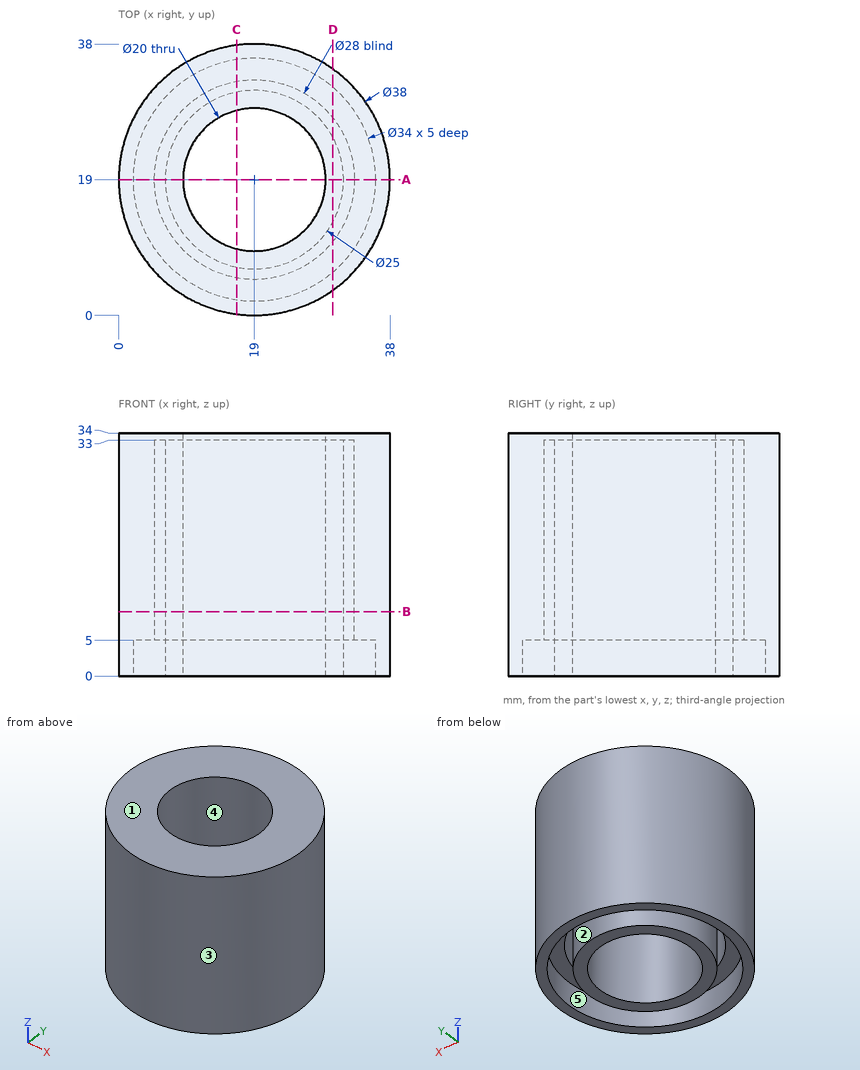
Drawing for the job (mm, zero at the part's lowest x, y, z). A direction names the side the tool comes from. Coordinates: 2 decimals unless noted, no trailing zeros. Order: outer loops, then holes, each group sorted by start corner. A loop starts at its lowest first (then second) coordinate and runs counter-clockwise, first axis right, second up. Notation, with made-up numbers: (-17.75, 64.25) - (29.25, 64.25) arc R36 ccw to (29.25, 102.25) - close; hole circle Ø10 at (-18.5, 9). An arc over 180 degrees is marked (long way). Use a Markdown table: item, result. Add a question column.
(1) Drill centre lines: line 1 along Y through (x, z) = (19, 10); line 2 along Y through (x, z) = (12, 24); line 3 along X through (y, z) = (23, 22). Where is each one in solid material? Low to high. Write a range as [from, to].
(2) Which spindle directions (+Z, -Z, +X, -X, +Y, -Y) get a long thin tool onto all of the face, cutting with end or side? Do the marked faces 4 and 5. Say none if no direction does.
(3) Saw through at D-D (x = 30). Give the cut face in (y, z).
(4) Saw through at C-C (x = 16.5). Give the cut face in (y, z), then the cut area to 3 significant figures.
(5) Pull direction Y, two halves, no side cores. Call the marked faces 1, 2 and 3: +Y half, -Y half, draft (parallel to the pull), parting line (faces both ways), or undercut.
(6) Flat gauge pins, fed straight in: pin 1 (1.5 mm diameter, centred on y = 15.5, z = 24.5, fed in from -X); pin 2 (5 mm diameter, centred on y = 8, z = 19.5, fed in from -X); pin 3 (5 mm diameter, centred on y = 10, z = 9.5, fed in from +X). Where does each tip first touch, or does it go through?
(7) Saw through at B-B (z = 9). Give the cut face in (x, y), then the cut area to 3 significant figures.
(8) Saw through at A-A (y = 19). Give the cut face in (x, z).
Solved:
| question | item | result |
|---|---|---|
| 1 | line 1 | y = [0, 5], [6.5, 9], [29, 31.5], [33, 38] |
| 1 | line 2 | y = [1.34, 6.88], [8.64, 11.86], [26.14, 29.36], [31.12, 36.66] |
| 1 | line 3 | x = [0.43, 5.58], [7.16, 9.83], [28.17, 30.84], [32.42, 37.57] |
| 2 | face 4 | +Z, -Z |
| 2 | face 5 | -Z |
| 3 | outline | (3.51, 0) - (6.04, 0) - (6.04, 5) - (10.34, 5) - (10.34, 33) - (13.06, 33) - (13.06, 0) - (24.94, 0) - (24.94, 33) - (27.66, 33) - (27.66, 5) - (31.96, 5) - (31.96, 0) - (34.49, 0) - (34.49, 34) - (3.51, 34) - close |
| 4 | outline | (0.17, 0) - (2.18, 0) - (2.18, 5) - (5.23, 5) - (5.23, 33) - (6.75, 33) - (6.75, 0) - (9.32, 0) - (9.32, 34) - (0.17, 34) - close; (28.68, 0) - (31.25, 0) - (31.25, 33) - (32.77, 33) - (32.77, 5) - (35.82, 5) - (35.82, 0) - (37.83, 0) - (37.83, 34) - (28.68, 34) - close |
| 4 | area | 491 mm² |
| 5 | face 1 | draft |
| 5 | face 2 | undercut |
| 5 | face 3 | parting line |
| 6 | pin 1 | stops at x = 0.2 |
| 6 | pin 2 | stops at x = 2.01 |
| 6 | pin 3 | stops at x = 36.85 |
| 7 | outline | circle Ø38 at (19, 19); circle Ø25 at (19, 19); hole circle Ø28 at (19, 19); hole circle Ø20 at (19, 19) |
| 7 | area | 695 mm² |
| 8 | outline | (0, 0) - (2, 0) - (2, 5) - (5, 5) - (5, 33) - (6.5, 33) - (6.5, 0) - (9, 0) - (9, 34) - (0, 34) - close; (29, 0) - (31.5, 0) - (31.5, 33) - (33, 33) - (33, 5) - (36, 5) - (36, 0) - (38, 0) - (38, 34) - (29, 34) - close |
